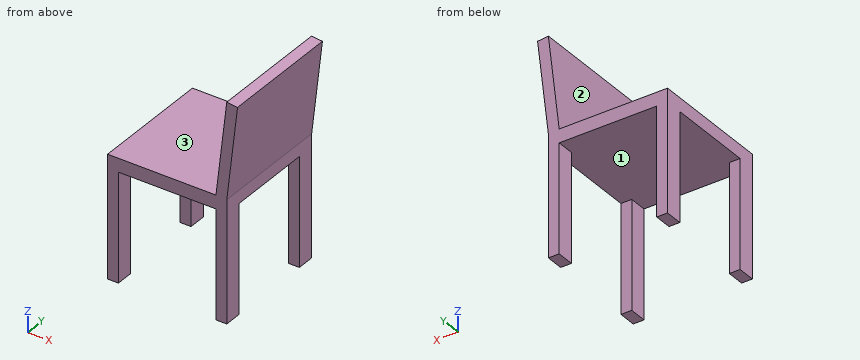
from build123d import *

# Parameters (mm, degrees)
F1_DEPTH      = 45
F2_W          = 31.9801214337
F2_H          = 40
F3_DEPTH      = 7.9751306906
F3_DEPTH_BACK = 40.001


with BuildPart() as f1:
    # F0 (on Front) → F1 (new body)
    with BuildSketch(Plane.XZ):
        Polygon((-4, 0), (0, 0), (0, 44.7721700924), (3.9741306906, 79.5458136354), (0, 80), (-4, 45), (-44, 45), (-44, 0), (-40, 0), (-40, 40), (-4, 40), align=None)
    extrude(amount=F1_DEPTH)

    # F2 (on face) → F3 (cut, two sides)
    with BuildSketch(Plane(origin=(-4, 0, 0), x_dir=(0, -1, 0), z_dir=(-1, 0, 0))) as f3_sk:
        with Locations((22.5, 20)):
            Rectangle(F2_W, F2_H)
    extrude(amount=-F3_DEPTH, mode=Mode.SUBTRACT)
    extrude(f3_sk.sketch, amount=F3_DEPTH_BACK, mode=Mode.SUBTRACT)


solid = f1.part
The listing builds one solid part. Answer for the finished solid, in the listing's coordinates (mm). Face numbers are marked on the shaded views. Coordinates: 2 decimals unless noted, no trailing zeros. Write each loop counter-clockwise with the first axis right and the second up, starting at its lowest first coordinate (ties: lowest second). Pieces come first, ordered by that corner, then holes. Notation, with made-up numbers: (-33.5, -11) - (-22.5, -11) arc R19 ccw to (-22.5, -1) - close; hole circle Ø11 at (32, 59). An arc over 180 degrees is marked (long way). Answer as CSV lines item,"result".
1. Find section D-D (z = 43). Give the vertices of the cut face in (x, y), plus the area to 3 significant figures.
Computed values:
outline,"(-44, -45) - (0, -45) - (0, 0) - (-44, 0) - close"
area,"1,980 mm²"
2. Find section B-B (x = -3). Give the vertices of the cut face in (y, z).
Computed values:
outline,"(-45, 0) - (-38.49, 0) - (-38.49, 40) - (-6.51, 40) - (-6.51, 0) - (0, 0) - (0, 53.75) - (-45, 53.75) - close"
3. Find section A-A (z = 33). Give the vertices of the cut face in (x, y).
Computed values:
outline,"(-44, -45) - (-40, -45) - (-40, -38.49) - (-44, -38.49) - close; (-44, -6.51) - (-40, -6.51) - (-40, 0) - (-44, 0) - close; (-4, -45) - (0, -45) - (0, -38.49) - (-4, -38.49) - close; (-4, -6.51) - (0, -6.51) - (0, 0) - (-4, 0) - close"
4. Straight lines are drawn through the part: line 1 (Y direction, x = -0.5, z = 19.5); line 2 (Z direction, x = -14, y = -19.5); line 3 (X direction, y = -25, z = 58.5). For each, find the intervals that lie inside material, in ascending order. Write a range as [from, to].
Computed values:
line 1,"y = [-45, -38.49], [-6.51, 0]"
line 2,"z = [40, 45]"
line 3,"x = [-2.46, 1.57]"
5. Determine the mould class of the marked faces 1, 2 and 3 for opening direction X: +X half, -X half, draft (parallel to the pull), parting line (faces both ways), or undercut.
Computed values:
face 1,"undercut"
face 2,"-X half"
face 3,"draft"
6. Given P1, Ø1.5, axis at x = -5, z = 46.5, coming from the +Y side; P2, Ø2, axis at y = -7, z = 55, coming from the +X side; P3, Ø8, axis at x = -8.5, y = -15, coming from the -Z side; P4, Ø7, axis at y = -4, z = 21, coming from the +X side, each flat-ended and moving along its own axis, determine where each tip first touches the part or whether it passes through.
Computed values:
P1,"passes through"
P2,"stops at x = 1.28"
P3,"stops at z = 40"
P4,"stops at x = 0"
7. Find section C-C (y = -21). Give the vertices of the cut face in (x, z), plus the area to 3 significant figures.
Computed values:
outline,"(-44, 40) - (0, 40) - (0, 44.77) - (3.97, 79.55) - (0, 80) - (-4, 45) - (-44, 45) - close"
area,"360 mm²"
